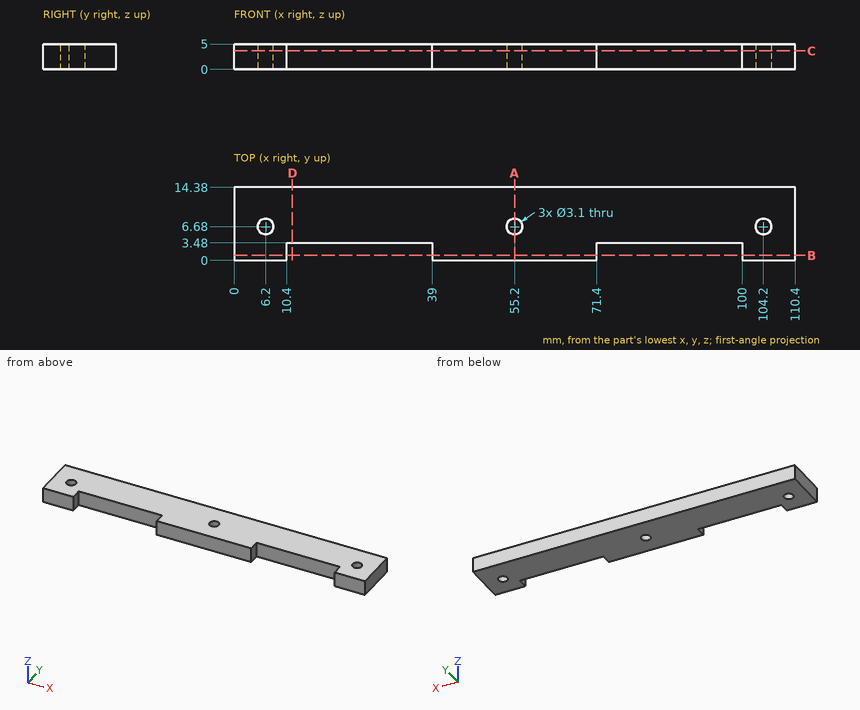
Job drawing, mm, ordinate dimensions from the low corner. One solid piece. Coordinates: 2 decimals unless noted, no trailing zeros. Order: outer loops, then holes, each group sorted by start corner. A loop starts at its lowest first (then second) coordinate and runs counter-clockwise, first axis right, second up. Notation, with made-up numbers: M 17.5,16.25 L 41.5,16.25 A20 cw 41.5,27.25 Z; hole C 11,41.25 d11. An arc over 180 degrees is marked long. Return JSON: item names as keys, results as strings.
1. Saw through at C-C (z = 3.65). Give the cut face in (x, y).
Ans:
{"outline": "M 0,0 L 10.4,0 L 10.4,3.48 L 39,3.48 L 39,0 L 71.4,0 L 71.4,3.48 L 100,3.48 L 100,0 L 110.4,0 L 110.4,14.38 L 0,14.38 Z; hole C 6.2,6.68 d3.1; hole C 55.2,6.68 d3.1; hole C 104.2,6.68 d3.1"}
2. Saw through at A-A (x = 55.2). Give the cut face in (y, z).
Ans:
{"outline": "M 0,0 L 5.13,0 L 5.13,5 L 0,5 Z; M 8.23,0 L 14.38,0 L 14.38,5 L 8.23,5 Z"}
3. Flat gauge pins, fed straight in: pin 1 (1.9 mm diameter, centred on x = 6.2, y = 6.68, fed in from -Z); pin 2 (1 mm diameter, centred on x = 75.5, z = 1, fed in from -Y). Where does each tip first touch, or does it go through?
Ans:
{"pin 1": "through", "pin 2": "y = 3.48"}
4. Drill centre lines: probe 1 along X at (y, z) = (0.5, 0.4); probe 2 along Y at (x, z) = (6, 1.3); probe 3 along X at (y, z) = (8, 4.05). Where is each one in solid material? Low to high.
Ans:
{"probe 1": "0 to 10.4, 39 to 71.4, 100 to 110.4", "probe 2": "0 to 5.14, 8.22 to 14.38", "probe 3": "0 to 5.39, 7.01 to 54.39, 56.01 to 103.39, 105.01 to 110.4"}
5. Saw through at B-B (y = 1). Give the cut face in (x, z).
Ans:
{"outline": "M 0,0 L 10.4,0 L 10.4,5 L 0,5 Z; M 39,0 L 71.4,0 L 71.4,5 L 39,5 Z; M 100,0 L 110.4,0 L 110.4,5 L 100,5 Z"}
6. Saw through at D-D (x = 11.5). Give the cut face in (y, z), and give its area (3 significant figures).
Ans:
{"outline": "M 3.48,0 L 14.38,0 L 14.38,5 L 3.48,5 Z", "area": "54.5 mm^2"}
